Autodesk Inventor part; units mm, degrees
ref_plane "YZ Plane" through (0, 0, 0) normal (1, 0, 0) x (0, 1, 0)
ref_plane "XZ Plane" through (0, 0, 0) normal (0, 1, 0) x (-1, 0, 0)
ref_plane "XY Plane" through (0, 0, 0) normal (0, 0, 1) x (1, 0, 0)
sketch "Sketch1" plane through (0, 0, 0) normal (0, 1, 0) x (-1, 0, 0)
  line L0 (0, 0) -> (-130, 0)
  line L1 (-130, 0) -> (-130, -20)
  line L2 (-130, -20) -> (0, -20)
  line L3 (0, -20) -> (0, 0)
  line L4 (0, -10) -> (-130, -10) construction
  line L5 (-46, 0) -> (-46, -20) construction
  line L6 (-84, 0) -> (-84, -20) construction
  line L7 (-65, 0) -> (-65, -20) construction
  line L8 (-39, 0) -> (-39, -20) construction
  line L9 (-91, 0) -> (-91, -20) construction
  circle A0 centre (-65, -10) radius 3
  line L10 (-20, 0) -> (-20, -20) construction
  line L11 (-110, 0) -> (-110, -20) construction
  circle A1 centre (-110, -10) radius 3
  circle A2 centre (-20, -10) radius 3
  dimension "d1" = 20
  dimension "d0" = 130
  dimension "d2" = 65
  dimension "d3" = 26
  dimension "d4" = 26
  dimension "d5" = 19
  dimension "d6" = 19
  dimension "d17" = 6
  dimension "d18" = 20
  dimension "d19" = 20
  dimension "d20" = 6
  dimension "d21" = 6
extrude "Extrusion1" add sketch "Sketch1" along normal blind 4
sketch "Sketch2" plane through (0, 4, 0) normal (0, 1, 0) x (1, 0, 0)
  line L0 (130, 20) -> (0, 20) construction
  line L1 (65, 20) -> (65, 0) construction
  line L2 (0, 0) -> (130, 0) construction
  line L3 (0, 20) -> (0, 0) construction
  line L4 (39, 20) -> (39, 0) construction
  line L5 (46, 20) -> (46, 0) construction
  line L6 (84, 20) -> (84, 0) construction
  line L7 (91, 20) -> (91, 0) construction
  line L8 (40.1, 20) -> (40.1, 0)
  line L9 (37.9, 20) -> (37.9, 0)
  line L10 (44.9, 20) -> (44.9, 0)
  line L11 (47.1, 20) -> (47.1, 0)
  line L12 (82.9, 20) -> (82.9, 0)
  line L13 (85.1, 20) -> (85.1, 0)
  line L14 (89.9, 20) -> (89.9, 0)
  line L15 (92.1, 20) -> (92.1, 0)
  line L16 (37.9, 20) -> (40.1, 20)
  line L17 (37.9, 0) -> (40.1, 0)
  line L18 (44.9, 0) -> (47.1, 0)
  line L19 (44.9, 20) -> (47.1, 20)
  line L20 (82.9, 20) -> (85.1, 20)
  line L21 (89.9, 20) -> (92.1, 20)
  line L22 (85.1, 0) -> (82.9, 0)
  line L23 (89.9, 0) -> (92.1, 0)
  dimension "d24" = 65
  dimension "d25" = 19
  dimension "d26" = 26
  dimension "d27" = 19
  dimension "d28" = 26
  dimension "d29" = 1.1
  dimension "d30" = 1.1
  dimension "d31" = 1.1
  dimension "d32" = 1.1
  dimension "d33" = 1.1
  dimension "d34" = 1.1
  dimension "d35" = 1.1
  dimension "d36" = 1.1
extrude "Extrusion2" cut sketch "Sketch2" against normal blind 3
properties part number "clamp"
Input: part model. Units: mm. Frame: model coordinates. A direction names the side the tool comes from. Give positions to 0.01 mm unless a question says otherwise; leave off trailing zeros. Order: outer loops, then holes, each group sorted by start corner. A loop starts at its lowest first (then second) coordinate and runs counter-clockwise, first axis right, second up. Notation, with made-up numbers: M -7,74.25 L 21,74.25 A9 ccw 21,89.25 Z; hole C 32.25,-38.75 d10. An arc over 180 degrees is marked long. One line per question, with ' | ' between items.
1) Section A-A on y = 2.3. Output: boundary loops of the cut face in (x, z).
Filled in:
outline: M 0,-20 L 37.9,-20 L 37.9,0 L 0,0 Z; M 40.1,-20 L 44.9,-20 L 44.9,0 L 40.1,0 Z; M 47.1,-20 L 82.9,-20 L 82.9,0 L 47.1,0 Z; M 85.1,-20 L 89.9,-20 L 89.9,0 L 85.1,0 Z; M 92.1,-20 L 130,-20 L 130,0 L 92.1,0 Z; hole C 20,-10 d6; hole C 65,-10 d6; hole C 110,-10 d6
2) Contact query for flat-ended pins moving along their axis: P1, Ø0.7, axis at x = 46.5, z = -6, coming from the +Y side; P2, Ø1.5, axis at y = 2.5, z = -12.5, coming from the -X side. Output: stop coordinate, or through.
Filled in:
P1: stops at y = 1 | P2: stops at x = 0
3) Section D-D on z = -3.5. Output: boundary loops of the cut face in (x, y), and give its area (3 significant figures).
Filled in:
outline: M 0,0 L 130,0 L 130,4 L 92.1,4 L 92.1,1 L 89.9,1 L 89.9,4 L 85.1,4 L 85.1,1 L 82.9,1 L 82.9,4 L 47.1,4 L 47.1,1 L 44.9,1 L 44.9,4 L 40.1,4 L 40.1,1 L 37.9,1 L 37.9,4 L 0,4 Z | area: 494 mm2
4) Ray query, L1, parallel to X at y = 3.7, z = -17.75; L2, parallel to Z at x = 110, y = 2.45; L3, parallel to X at y = 0.5, z = -12.75. Return the intervals inside material, ascending.
Filled in:
L1: x = 0 to 37.9, 40.1 to 44.9, 47.1 to 82.9, 85.1 to 89.9, 92.1 to 130 | L2: z = -20 to -13, -7 to 0 | L3: x = 0 to 18.8, 21.2 to 63.8, 66.2 to 108.8, 111.2 to 130
5) Draft query along Z for faces 3 (the face through (67.4, 2, -8.2)), 4 (the face through (64, 2, 0)), 5 (the face through (37.9, 3, -10)). Return one class per face: pulls with the +Z half, pulls with the -Z half, needs draft (parallel to the pull), parting line crosses it, or undercut.
Filled in:
face 3: undercut | face 4: pulls with the +Z half | face 5: needs draft
6) Section B-B on z = -10. State how many separate pieces and enclosed holes the cut face has, and give its area (3 significant figures).
Filled in:
separate pieces: 4 | enclosed holes: 0 | area: 422 mm2
7) Access query for faces 1 (the face through (88, 4, -10)), 2 (the face through (44.9, 3, -10)). Directions: +Z, -Z, +X, -X, +Y, -Y. A direction counts if a zero-diameter tool reaches every point of the face in a straight line with its end or side. Return the directions, or none.
Filled in:
face 1: +Z, -Z, +X, -X, +Y | face 2: +Z, -Z, +Y
8) Section C-C on x = 108.5. Output: boundary loops of the cut face in (y, z).
Filled in:
outline: M 0,-20 L 4,-20 L 4,-12.6 L 0,-12.6 Z; M 0,-7.4 L 4,-7.4 L 4,0 L 0,0 Z
